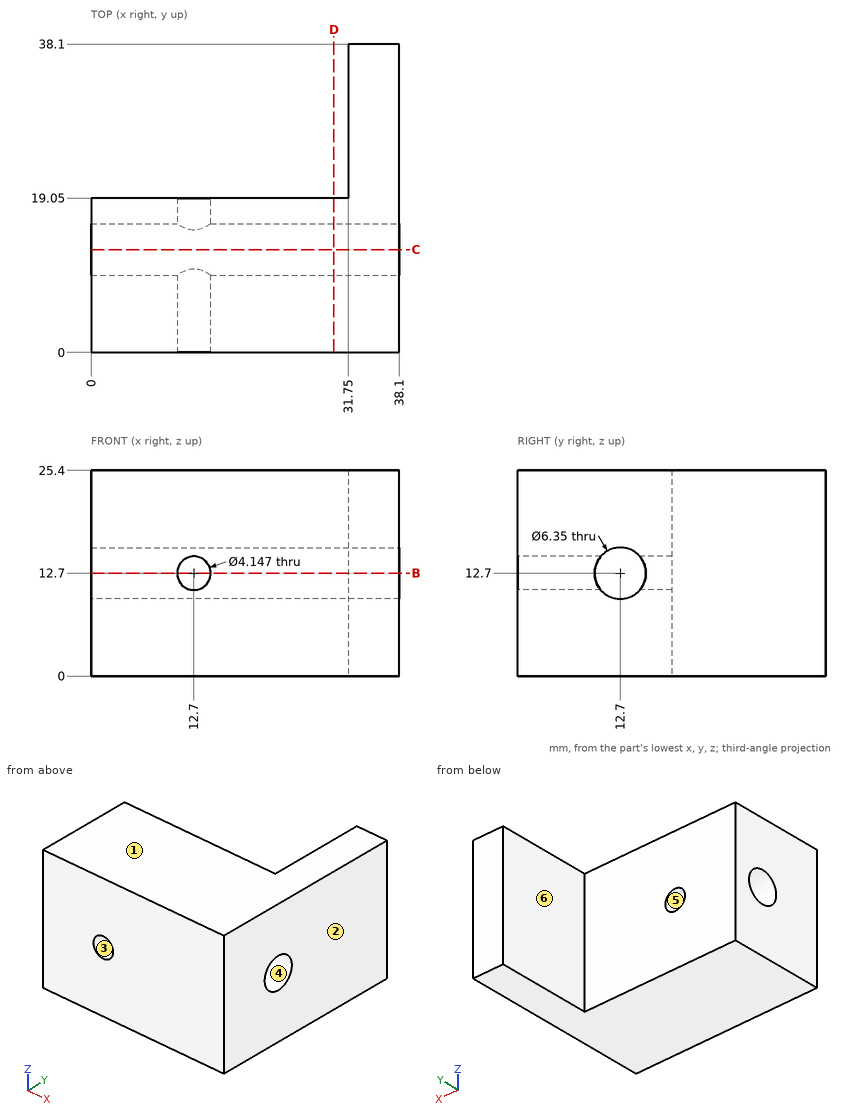
Job drawing, mm, ordinate dimensions from the low corner. One solid piece. A direction names the side the tool comes from. Coordinates: 2 decimals unless noted, no trailing zeros. Order: outer loops, then holes, each group sorted by start corner. A loop starts at its lowest first (then second) coordinate and runs counter-clockwise, first axis right, second up. Notation, with made-up numbers: (62.25, 23) -> (114.25, 23) arc R26 cw to (114.25, 57) -> close; hole circle Ø4 at (-11, 0.5). An arc over 180 degrees is marked (long way). Put each result on its own line as item: value. Start each with the question number.
(1) Which spindle directions (+Z, -Z, +X, -X, +Y, -Y) get a long thin tool onto all of the face, cutting with end or side? Do the marked faces 5 and 6. Say none if no direction does.
(2) Mould opens along Z. For the marked faces 1, 2, 3 and 4 say: pulls with the +Z half, pulls with the -Z half, needs draft (parallel to the pull), parting line crosses it, or undercut.
(3) Probe line 1 along Y through (x, z) = (25, 12.7) (3 decimals); line 2 along X through (y, z) = (4.75, 12.7); line 3 along Z through (x, y) = (12.7, 17.75). List the from-to ranges inside material, lowest first. Write a range as [from, to].
(4) Band-saw the part on B-B (z = 12.7). Count the separate pieces of the cut face and the enclosed holes in it, then the cut area to 3 significant figures.
(5) Band-saw the part on C-C (y = 12.7). Give the cut face in (x, z) (3 decimals), then the cut area to 3 significant figures.
(6) Band-saw the part on D-D (x = 30). Give the cut face in (y, z) (3 decimals), then the cut area to 3 significant figures.
(7) Pin check, flat tip, straight feed: pin 1 Ø4 at (x, z) = (6.5, 16) entering from +Y. Stop position of the tip, or through.
Determined:
1. face 5: +Y, -Y
1. face 6: +Z, -Z, -X, +Y
2. face 1: pulls with the +Z half
2. face 2: needs draft
2. face 3: undercut
2. face 4: undercut
3. line 1: y = [0, 9.525], [15.875, 19.05]
3. line 2: x = [0, 10.63], [14.77, 38.1]
3. line 3: z = [0, 10.63], [14.77, 25.4]
4. separate pieces: 4
4. enclosed holes: 0
4. area: 552 mm²
5. outline: (0, 0) -> (38.1, 0) -> (38.1, 9.525) -> (0, 9.525) -> close; (0, 15.875) -> (38.1, 15.875) -> (38.1, 25.4) -> (0, 25.4) -> close
5. area: 726 mm²
6. outline: (0, 0) -> (19.05, 0) -> (19.05, 25.4) -> (0, 25.4) -> close; hole circle Ø6.35 at (12.7, 12.7)
6. area: 452 mm²
7. pin 1: stops at y = 19.05
